Verification items for the finished model (mm, model axes). Face numbers are marked on the shaded views. A direction names the side the tool comes from. Give positions to 0.01 mm unless a question says otherwise; leave off trailing zeros. Loops run counter-clockwise (first coordinate to the right, second up) from the corner with the lowest first, then second, coordinate; pieces in that order, holes last. Notation, with made-up numbers: M 13.25,74.5 L 26.25,74.5 A18 cw 26.25,102.5 Z; hole C 73,51 d8. An arc over 180 degrees is marked long. Use a Markdown table: item, result.
from build123d import *

# Parameters (mm, degrees)
F0_R     = 70
F1_DEPTH = 59
F2_R     = 70
F2_R_2   = 61
F3_DEPTH = 25
F4_R     = 36
F5_DEPTH = 59
F6_R     = 44
F7_DEPTH = 16


with BuildPart() as f1:
    # F0 (on Front) → F1 (new body)
    with BuildSketch(Plane.XZ):
        Circle(F0_R)
    extrude(amount=-F1_DEPTH)

    # F2 (on face) → F3 (cut)
    with BuildSketch(Plane.XZ):
        Circle(F2_R)
        Circle(F2_R_2, mode=Mode.SUBTRACT)
    extrude(amount=-F3_DEPTH, mode=Mode.SUBTRACT)

    # F4 (on face) → F5 (cut, through all)
    with BuildSketch(Plane.XZ):
        Circle(F4_R)
    extrude(amount=-F5_DEPTH, mode=Mode.SUBTRACT)

    # F6 (on face) → F7 (cut)
    with BuildSketch(Plane(origin=(0, 59, 0), x_dir=(-1, 0, 0), z_dir=(0, 1, 0))):
        with Locations((-3.819107, 0)):
            Circle(F6_R)
    extrude(amount=-F7_DEPTH, mode=Mode.SUBTRACT)


solid = f1.part
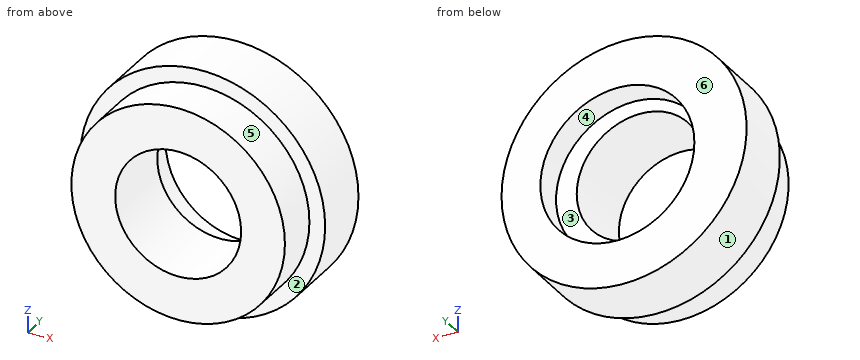
(1) Material ranges on line 1 (Z direction, x = 0, y = 29); line 2 (Y direction, x = 34.5, z = 17); line 3 (X direction, y = 26, z = 60), recorded low to high.
Results below:
| item | result |
|---|---|
| line 1 | -70 to -36, 36 to 70 |
| line 2 | 0 to 43 |
| line 3 | -36.06 to 36.06 |
(2) Cross-section at A-A on z = 0. Record the cut outline in (x, y).
Results below:
| item | result |
|---|---|
| outline | M -70,25 L -61,25 L -61,0 L -36,0 L -36,43 L -40.18,43 L -40.18,59 L -70,59 Z; M 36,0 L 61,0 L 61,25 L 70,25 L 70,59 L 47.82,59 L 47.82,43 L 36,43 Z |
(3) Cross-section at B-B on x = 15.5. Record the cut outline in (y, z), then the cut area to 3 significant figures.
Results below:
| item | result |
|---|---|
| outline | M 0,-59 L 25,-59 L 25,-68.26 L 59,-68.26 L 59,-42.42 L 43,-42.42 L 43,-32.49 L 0,-32.49 Z; M 0,32.49 L 43,32.49 L 43,42.42 L 59,42.42 L 59,68.26 L 25,68.26 L 25,59 L 0,59 Z |
| area | 3,440 mm^2 |
(4) Gauge pin test, flat ends, axial feed: P1, Ø6, axis at x = 52, y = 42, coming from the -Z side; P2, Ø6, axis at y = 45, z = -33, coming from the +X side; P3, Ø5, axis at x = 31, y = 14, coming from the +Z side. Record the tip position at first contact, or that the pin passes through.
Results below:
| item | result |
|---|---|
| P1 | z = -49.99 |
| P2 | x = 63.25 |
| P3 | z = 53.93 |
(5) Cross-section at D-D on z = 54.5. Record the cut outline in (x, y), then the cut area to 3 significant figures.
Results below:
| item | result |
|---|---|
| outline | M -43.93,25 L -27.4,25 L -27.4,0 L 27.4,0 L 27.4,25 L 43.93,25 L 43.93,59 L -43.93,59 Z |
| area | 4,360 mm^2 |
(6) Draft check along Z on the marked faces 1, 2 and 3. Enter one of: +Z half, -Z half, draft (parallel to the pull), parting line (faces both ways), or undercut.
Results below:
| item | result |
|---|---|
| face 1 | parting line |
| face 2 | draft |
| face 3 | undercut |
(7) Set-up check for the marked faces 4, 5 and 6: record each of +Z, -Z, +X, -X, +Y, -Y from which the full face is reachable in a straight line by a thin tool's end or side.
Results below:
| item | result |
|---|---|
| face 4 | +Y |
| face 5 | -Y |
| face 6 | +Z, -Z, +X, -X, +Y |
(8) Cross-section at C-C on y = 41. Record the cut outline in (x, z).
Results below:
| item | result |
|---|---|
| outline | C 0,0 d140; hole C 0,0 d72 |
